For this review, take the finished solid that the model builds, in its own axes (mm). Face numbers are marked on the shaded views. A direction names the side the tool comes from. Give positions to 0.01 mm unless a question says otherwise; leave off trailing zeros. Loops run counter-clockwise (first coordinate to the right, second up) from the corner with the lowest first, then second, coordinate; pieces in that order, holes last.
```python
from build123d import *

# Parameters (mm, degrees)
F0_R        = 112.954685
F0_R_2      = 90.326171
F1_DEPTH    = 175
F1_FACE_R   = 112.954685
F1_FACE_R_2 = 90.326171
F2_DEPTH    = 87
F3_W        = 293.390907
F3_H        = 287.415445
F4_DEPTH    = 25


with BuildPart() as f1:
    # F0 (on Top) → F1 (new body)
    with BuildSketch(Plane.XY):
        with Locations((29.057469, 144.334614)):
            Circle(F0_R)
        with Locations((29.057469, 144.334614)):
            Circle(F0_R_2, mode=Mode.SUBTRACT)
    extrude(amount=F1_DEPTH)

    # F1_face (on face) → F2 (join)
    with BuildSketch(Plane(origin=(29.057469, 144.334614, 175), x_dir=(1, 0, 0), z_dir=(0, 0, 1))):
        Circle(F1_FACE_R)
        Circle(F1_FACE_R_2, mode=Mode.SUBTRACT)
    extrude(amount=F2_DEPTH)

    # F3 (on Top) → F4 (join)
    with BuildSketch(Plane.XY):
        with Locations((32.84381, 143.707722)):
            Rectangle(F3_W, F3_H)
    extrude(amount=F4_DEPTH)


solid = f1.part
```
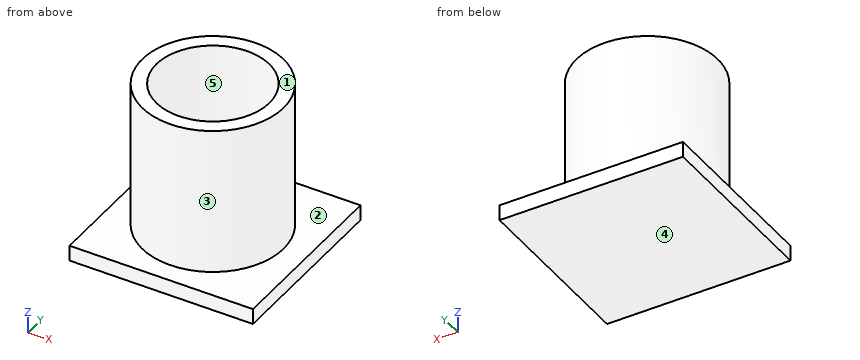
Item 1: Take a section at A-A on y = 116. Give the boundary of the cut face in (x, z), and give its area (3 significant figures).
Answer:
outline: (-113.85, 0) - (179.54, 0) - (179.54, 25) - (138.4, 25) - (138.4, 262) - (114.82, 262) - (114.82, 25) - (-56.71, 25) - (-56.71, 262) - (-80.29, 262) - (-80.29, 25) - (-113.85, 25) - close
area: 18,500 mm2
Item 2: The part is to be moulded in two halves that separate along X. For the marked faces 3, 4 and 5, say which applies: released by +X, released by -X, zero draft, split by the parting line, or undercut.
Answer:
face 3: split by the parting line
face 4: zero draft
face 5: undercut
Item 3: Tool access review of the marked faces 1 and 2: name each direction out of +Z, -Z, +X, -X, +Y, -Y from which nothing blocks a thin tool from reaching the whole face with its end or side.
Answer:
face 1: +Z, +X, -X, +Y, -Y
face 2: +Z
Item 4: Take a section at C-C on z = 85.5. Give the boundary of the cut face in (x, y), and give its area (3 significant figures).
Answer:
outline: circle Ø225.91 at (29.06, 144.33); hole circle Ø180.65 at (29.06, 144.33)
area: 14,500 mm2
Item 5: Clearance check with flat-ended pins moving along their axes: pin 1 Ø5 at (y, z) = (148, 132) entering from -X; pin 2 Ø4 at (x, y) = (20.5, 150) entering from +Z; pin 3 Ø10 at (x, z) = (62.5, 43) entering from -Y. State where each tip first meets the part, or that it passes through.
Answer:
pin 1: stops at x = -83.89
pin 2: stops at z = 25
pin 3: stops at y = 35.02
Item 6: Take a section at B-B on x = 132. Give the boundary of the cut face in (y, z).
Answer:
outline: (0, 0) - (287.42, 0) - (287.42, 25) - (190.83, 25) - (190.83, 262) - (97.84, 262) - (97.84, 25) - (0, 25) - close
Item 7: Take a section at D-D on y = 152. Give the boundary of the cut face in (x, z), and give its area (3 significant figures).
Answer:
outline: (-113.85, 0) - (179.54, 0) - (179.54, 25) - (141.75, 25) - (141.75, 262) - (119.06, 262) - (119.06, 25) - (-60.94, 25) - (-60.94, 262) - (-83.64, 262) - (-83.64, 25) - (-113.85, 25) - close
area: 18,100 mm2
Item 8: For L1, parallel to X at y = 148, z = 81; L2, parallel to Z at x = -62, y = 34; L3, parallel to X at y = 228, z = 220.5, list the stretches that pass through material, from the lowest coordinate up.
Answer:
L1: x = -83.84 to -61.19, 119.31 to 141.95
L2: z = 0 to 25
L3: x = -46.83 to -4.99, 63.1 to 104.94
